Work out the finished part from the listing and answer in its coordinate system (mm). Face numbers are marked on the shaded views. A direction names the side the tool comes from. Round coordinates to 2 decimals unless told otherwise and drop trailing zeros. Write each loop counter-clockwise with the first axis right and the second up, starting at its lowest first coordinate (ties: lowest second). Pieces come first, ordered by that corner, then holes. Notation, with made-up numbers: M 69,20.25 L 100,20.25 A14 cw 100,25.25 Z; hole C 14,62 d2. An arc over 180 degrees is marked long. One line per item, written item: value. Start each with the question number.
Q1. Find section A-A (y = 15). Write down the section's boundary in (x, z).
Q2. A tool of negligible diameter and unlimited length cuts with its end or side. For the marked faces 1 and 2, from which of +Z, -Z, +X, -X, +Y, -Y can it reach the whole face along a straight path? Write none if from no direction.
Q3. Given pin 1 Ø9 at (x, y) = (-82.5, 21) entering from +Z, flat-ended and moving along its own axis, determine where the tip first touches the part or whether it passes through.
Q4. Find section C-C (x = -30). Write down the section's boundary in (y, z), and give its area (3 significant figures).
Q5. Find section B-B (z = -141). Write down the section's boundary in (x, y).
Q6. The mould has two halves that part along X. Classify the marked faces 3, 4, 5 and 6: released by +X, released by -X, zero draft, split by the parting line, or undercut.
Q7. Consider probe 1 along Z at (x, y) = (-46, 18.5); probe 2 along X at (y, z) = (20.5, -102); probe 3 along Y at (x, z) = (-87, -212). Determine where each line is inside the solid, lowest interval first.
Autodesk Inventor part; units mm, degrees
ref_plane "YZ Plane" through (0, 0, 0) normal (1, 0, 0) x (0, 1, 0)
ref_plane "XZ Plane" through (0, 0, 0) normal (0, 1, 0) x (-1, 0, 0)
ref_plane "XY Plane" through (0, 0, 0) normal (0, 0, 1) x (1, 0, 0)
sketch "Boceto1" plane through (0, 0, 0) normal (0, 1, 0) x (-1, 0, 0)
  line L0 (0, 0) -> (140, 0)
  line L1 (140, 0) -> (140, -245)
  line L2 (140, -245) -> (0, -245)
  line L3 (0, -245) -> (0, 0)
  dimension "d0" = 140
  dimension "d1" = 245
extrude "Extrusión1" add sketch "Boceto1" along normal blind 50
sketch "Boceto2" plane through (0, 0, 0) normal (0, -1, 0) x (1, 0, 0)
  line L0 (0, -245) -> (-140, -245)
  line L1 (0, 0) -> (0, -245)
  line L2 (-140, 0) -> (0, 0)
  line L3 (-140, -245) -> (-140, 0)
  line L4 (29.1712, 0) -> (29.1712, -20)
  line L5 (0, 50.4533) -> (-20, 50.4533)
  line L6 (-175.5774, 0) -> (-175.5774, -20)
  line L7 (-175.5774, -245) -> (-175.5774, -225)
  line L8 (29.1712, -245) -> (29.1712, -225)
  line L9 (0, -265) -> (-20, -265)
  line L10 (-140, 34.3082) -> (-120, 34.3082)
  line L11 (-140, -269.5122) -> (-120, -269.5122)
  line L12 (-20, -20) -> (-120, -20)
  line L13 (-120, -20) -> (-120, -225)
  line L14 (-120, -225) -> (-20, -225)
  line L15 (-20, -225) -> (-20, -20)
  dimension "d4" = 20
  dimension "d5" = 20
  dimension "d7" = 20
  dimension "d9" = 20
  dimension "d10" = 20
  dimension "d11" = 20
  dimension "d12" = 20
  dimension "d13" = 20
extrude "Extrusión2" cut sketch "Boceto2" against normal blind 30 contours L15 L14 L13 L12
properties part number "Lamina Superior"
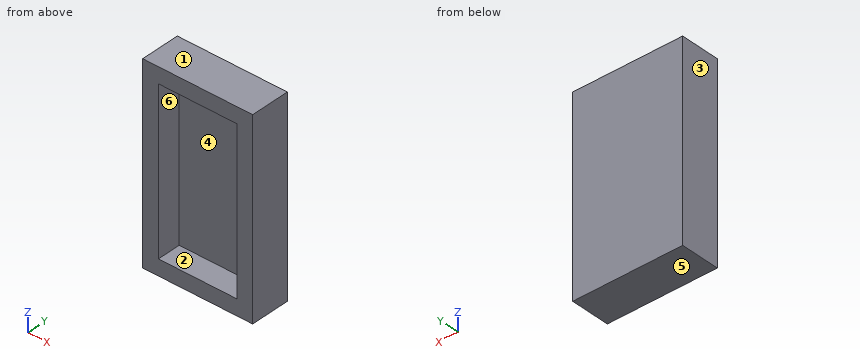
The answers:
1. outline: M -140,-245 L 0,-245 L 0,0 L -140,0 Z; hole M -120,-225 L -20,-225 L -20,-20 L -120,-20 Z
2. face 1: +Z, +X, -X, +Y, -Y
2. face 2: -Y
3. pin 1: z = 0
4. outline: M 0,-245 L 50,-245 L 50,0 L 0,0 L 0,-20 L 30,-20 L 30,-225 L 0,-225 Z
4. area: 6,100 mm2
5. outline: M -140,0 L -120,0 L -120,30 L -20,30 L -20,0 L 0,0 L 0,50 L -140,50 Z
6. face 3: released by -X
6. face 4: undercut
6. face 5: zero draft
6. face 6: undercut
7. probe 1: -245 to -225, -20 to 0
7. probe 2: -140 to -120, -20 to 0
7. probe 3: 30 to 50
